Geometry: see drawing. Coordinates: mm, zero at the bounding-box minimum. A direction names the side the tool comes from. Round coordinates to 2 decimals unless told otherwise and drop trailing zeros. Loops run counter-clockwise (first coordinate to the right, second up) from the corner with the lowest first, then second, coordinate; pieces in that order, holes last.
(1) Access query for the marked faces 1 and 2. Directions: +Z, -Z, +X, -X, +Y, -Y. A direction counts if a zero-diameter tool reaches every point of the face in a straight line with its end or side. Return the directions, or none.
(2) Cut plane D-D, the plane x = 18.5. Output: boundary loops of the cut face in (y, z) (1 decimal).
(3) Line query: line 1 (Y direction, x = 30.3, z = 65); line 2 (Y direction, x = 8, z = 57.5) (1 decimal); line 3 (Y direction, x = 30, z = 15). Output: solid intervals per line, ascending.
(4) First-contact query: pin 1 Ø2 at (y, z) = (12.5, 44.5) entering from -X (1 decimal); pin 2 Ø1.5 at (x, z) = (16.5, 70.5) entering from +Y (1 decimal); pin 3 Ø10 at (y, z) = (9, 9) entering from -X (1 decimal). Flat tips, straight axial feed; report the tip coordinate or a pass-through.
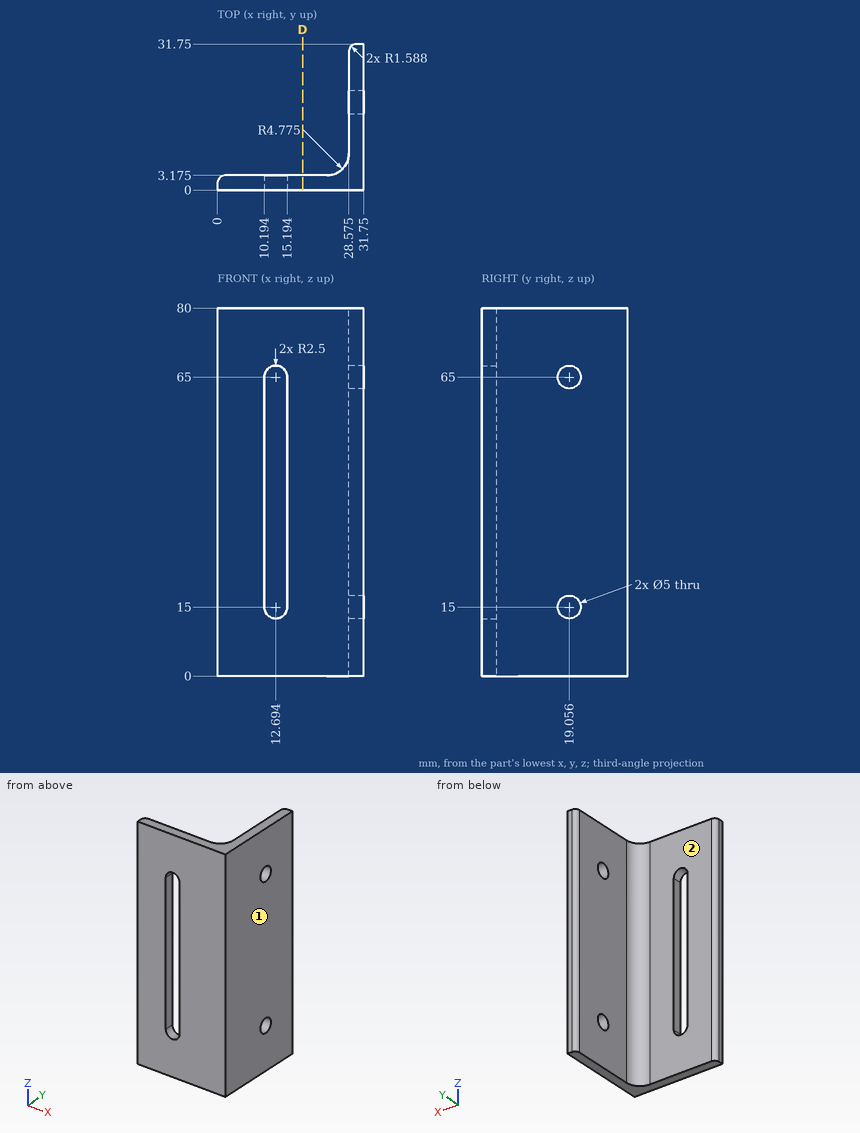
Reported:
1. face 1: +Z, -Z, +X, +Y, -Y
1. face 2: +Z, -Z, -X, +Y
2. outline: (0, 0) - (3.2, 0) - (3.2, 80) - (0, 80) - close
3. line 1: y = 0 to 16.56, 21.56 to 31.75
3. line 2: y = 0 to 3.2
3. line 3: y = 0 to 16.56, 21.56 to 31.74
4. pin 1: stops at x = 28.6
4. pin 2: stops at y = 3.2
4. pin 3: stops at x = 26.5
